Can you work these out from the drawing? Everything is in mm from the part's minimum corner. Give positions to 0.01 mm unless a question says otherwise; leave off trailing zeros. Order: outer loops, then holes, each group sorted by start corner. A loop starts at its lowest first (then second) coordinate and runs counter-clockwise, first axis right, second up. Notation, with made-up numbers: (-1.5, 85.5) -> (32.5, 85.5) arc R34 cw to (32.5, 120.5) -> close; hole circle Ø7 at (6.25, 88.25). An arc over 180 degrees is marked (long way). One line per item, written item: value.
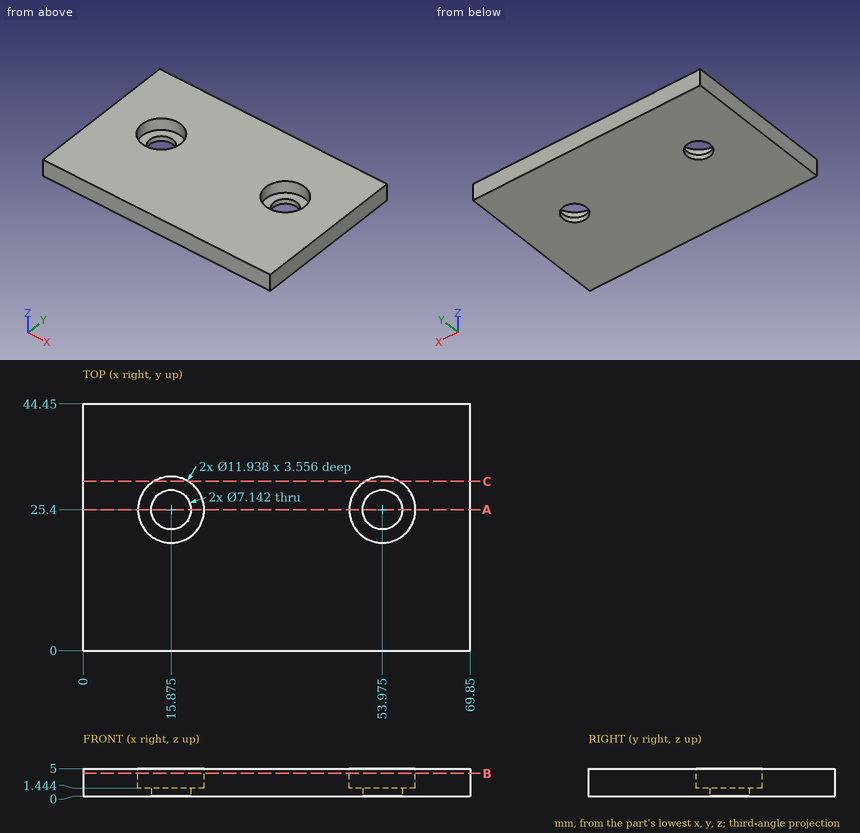
1) For P1, Ø11.5, axis at x = 53.975, y = 25.4, coming from the +Z side, with a flat end and sliding along its axis, tell me the tip position at first contact or that it passes through.
Answer below:
P1: stops at z = 1.44
2) If I drill on line 1 along X through (y, z) = (23, 2.9); line 2 along X through (y, z) = (27.5, 4.4); line 3 along Y through (x, z) = (54, 4), over which ranges is the centre line in solid material (lowest first)?
Answer below:
line 1: x = 0 to 10.41, 21.34 to 48.51, 59.44 to 69.85
line 2: x = 0 to 10.29, 21.46 to 48.39, 59.56 to 69.85
line 3: y = 0 to 19.43, 31.37 to 44.45
3) Suppose I cut it at A-A, the plane y = 25.4. Write out the boundary of the cut face in (x, z).
Answer below:
outline: (0, 0) -> (12.3, 0) -> (12.3, 1.44) -> (9.91, 1.44) -> (9.91, 5) -> (0, 5) -> close; (19.45, 0) -> (50.4, 0) -> (50.4, 1.44) -> (48.01, 1.44) -> (48.01, 5) -> (21.84, 5) -> (21.84, 1.44) -> (19.45, 1.44) -> close; (57.55, 0) -> (69.85, 0) -> (69.85, 5) -> (59.94, 5) -> (59.94, 1.44) -> (57.55, 1.44) -> close
4) Suppose I cut it at B-B, the plane z = 4.15. State how many separate pieces and enclosed holes the cut face has, then the cut area to 3 significant figures.
Answer below:
separate pieces: 1
enclosed holes: 2
area: 2,880 mm2
5) Suppose I cut it at C-C, the plane y = 30.5. Write out the boundary of the cut face in (x, z), then the cut area to 3 significant figures.
Answer below:
outline: (0, 0) -> (69.85, 0) -> (69.85, 5) -> (57.08, 5) -> (57.08, 1.44) -> (50.87, 1.44) -> (50.87, 5) -> (18.98, 5) -> (18.98, 1.44) -> (12.77, 1.44) -> (12.77, 5) -> (0, 5) -> close
area: 305 mm2
